from build123d import *

# Parameters (mm, degrees)
SKETCH1_W           = 18
SKETCH1_H           = 6
BOSS_EXTRUDE1_DEPTH = 17.5
SKETCH2_R           = 1.5
CUT_EXTRUDE1_DEPTH  = 20.906029237
FILLET1_R           = 2
BOSS_EXTRUDE2_DEPTH = 3.75
SKETCH4_W           = 4.2
SKETCH4_H           = 4
BOSS_EXTRUDE3_DEPTH = 2.25
SKETCH5_W           = 4.2
SKETCH5_H           = 8.25
CUT_EXTRUDE2_DEPTH  = 1.25
FILLET5_R           = 1
FILLET6_R           = 1.5
FILLET7_R           = 0.75


with BuildPart() as part:
    # Sketch1 → Boss-Extrude1 (new body)
    with BuildSketch(Plane(origin=(0, 0, 0), x_dir=(1, 0, 0), z_dir=(0, 1, 0))):
        Rectangle(SKETCH1_W, SKETCH1_H)
    extrude(amount=BOSS_EXTRUDE1_DEPTH)

    # Sketch2 → Cut-Extrude1 (cut, through all)
    with BuildSketch(Plane(origin=(0, 17.5, 0), x_dir=(1, 0, 0), z_dir=(0, 1, 0))):
        with Locations(Location((-5, 0, 0), (0, 0, 270))):
            Circle(SKETCH2_R)
        with Locations(Location((5, 0, 0), (0, 0, 90))):
            Circle(SKETCH2_R)
    extrude(amount=-CUT_EXTRUDE1_DEPTH, mode=Mode.SUBTRACT)

    # Fillet1
    fillet1_edges = [part.edges().sort_by_distance(p)[0] for p in [
        (9, 8.75, 3),
        (-9, 8.75, 3),
        (-9, 8.75, -3),
        (9, 8.75, -3),
    ]]
    fillet(fillet1_edges, radius=FILLET1_R)

    # Sketch3 → Boss-Extrude2 (add)
    with BuildSketch(Plane(origin=(0, 0, -3), x_dir=(-1, 0, 0), z_dir=(0, 0, -1))):
        Polygon((-3.25, 17.5), (-3.25, 13), (3.25, 13), (3.25, 17.5), (2.1, 17.5), (2.1, 13.5), (-2.1, 13.5), (-2.1, 17.5), align=None)
    extrude(amount=BOSS_EXTRUDE2_DEPTH)

    # Sketch4 → Boss-Extrude3 (add)
    with BuildSketch(Plane(origin=(0, 0, -3), x_dir=(-1, 0, 0), z_dir=(0, 0, -1))):
        with Locations((0, 15.5)):
            Rectangle(SKETCH4_W, SKETCH4_H)
    extrude(amount=BOSS_EXTRUDE3_DEPTH)

    # Sketch5 → Cut-Extrude2 (cut)
    with BuildSketch(Plane(origin=(0, 17.5, 0), x_dir=(1, 0, 0), z_dir=(0, 1, 0))):
        with Locations((0, 1.125)):
            Rectangle(SKETCH5_W, SKETCH5_H)
    extrude(amount=-CUT_EXTRUDE2_DEPTH, mode=Mode.SUBTRACT)

    # Fillet5
    fillet5_edges = [part.edges().sort_by_distance(p)[0] for p in [
        (0, 16.25, 3),
        (0, 16.25, -5.25),
    ]]
    fillet(fillet5_edges, radius=FILLET5_R)

    # Fillet6
    fillet6_edges = [part.edges().sort_by_distance(p)[0] for p in [
        (0, 13, -3),
        (-3.25, 15.25, -3),
        (3.25, 15.25, -3),
    ]]
    fillet(fillet6_edges, radius=FILLET6_R)

    # Fillet7
    # the kernel refuses this fillet: 0.75 mm, written as the material it takes off along each edge
    with BuildSketch(Plane(origin=(5.125, 13, -6.75), x_dir=(0, 1, 0), z_dir=(-1, 0, 0))) as fillet7_piece_1:
        with BuildLine():
            CenterArc((FILLET7_R, -FILLET7_R), FILLET7_R, 90, 90)
            Line((0, -FILLET7_R), (0, 0))
            Line((0, 0), (FILLET7_R, 0))
        make_face()
    extrude(amount=10.25, mode=Mode.SUBTRACT)


solid = part.part
Geometry: final body of the model. Coordinates: model frame, mm. A direction names the side the tool comes from. Round coordinates to 2 decimals unless told otherwise and drop trailing zeros. Loops run counter-clockwise (first coordinate to the right, second up) from the corner with the lowest first, then second, coordinate; pieces in that order, holes last. Notation, with made-up numbers: M -7,56 L 39,56 A28 ccw 39,76 Z; hole C 41.5,79 d5. An arc over 180 degrees is marked long. One line per question, with ' | ' between items.
(1) Pull-direction query (X, two-part tool) for faces 4 (the cylindrical face through (-8.43, 8.87, 2.4)), 5 (the flat face through (0, 13, -5)), 6 (the flat face through (0, 13.5, -6)); classes: +X half, -X half, draft (parallel to the pull), parting line (faces both ways), or undercut.
Check result:
face 4: -X half | face 5: draft | face 6: undercut
(2) Cut plane C-C on z = 0. Return the cut outline in (x, y), plus the area to 3 significant figures.
Check result:
outline: M -9,0 L -6.5,0 L -6.5,17.5 L -9,17.5 Z; M -3.5,0 L 3.5,0 L 3.5,17.5 L 2.1,17.5 L 2.1,16.25 L -2.1,16.25 L -2.1,17.5 L -3.5,17.5 Z; M 6.5,0 L 9,0 L 9,17.5 L 6.5,17.5 Z | area: 205 mm2
(3) Cut plane A-A on x = -5. Return the cut outline in (y, z).
Check result:
outline: M 0,-3 L 17.5,-3 L 17.5,-1.5 L 0,-1.5 Z; M 0,1.5 L 17.5,1.5 L 17.5,3 L 0,3 Z
(4) Material intervals for line 1 along X through (y, z) = (4, 0); line 2 along Z through (x, y) = (5, 5.5); line 3 along X through (y, z) = (15.25, -0.5), sorted ascending. Write a range as from..to.
Check result:
line 1: x = -9..-6.5, -3.5..3.5, 6.5..9 | line 2: z = -3..-1.5, 1.5..3 | line 3: x = -9..-6.41, -3.59..3.59, 6.41..9
(5) Cut plane B-B on y = 14.5. Return the cut outline in (x, z).
Check result:
outline: M -9,-1 A2 ccw -7,-3 L -4.75,-3 A1.5 cw -3.25,-4.5 L -3.25,-6.75 L -2.1,-6.75 L -2.1,-5.25 L 2.1,-5.25 L 2.1,-6.75 L 3.25,-6.75 L 3.25,-4.5 A1.5 cw 4.75,-3 L 7,-3 A2 ccw 9,-1 L 9,1 A2 ccw 7,3 L -7,3 A2 ccw -9,1 Z; hole C -5,0 d3; hole C 5,0 d3
(6) Contact query for flat-ended pins moving along their axis: P1, Ø2.5, axis at y = 15.5, z = -5, coming from the -X side; P2, Ø2.5, axis at x = -5, z = 0, coming from the +Y side; P3, Ø8, axis at x = -1.5, y = 5.5, coming from the -Z side; P4, Ø0.8, axis at x = -0.5, z = -5.5, coming from the -Y side. Output: stop coordinate, or through.
Check result:
P1: stops at x = -3.45 | P2: passes through | P3: stops at z = -3 | P4: stops at y = 13
(7) Cut plane D-D on y = 7. Return the cut outline in (x, z).
Check result:
outline: M -9,-1 A2 ccw -7,-3 L 7,-3 A2 ccw 9,-1 L 9,1 A2 ccw 7,3 L -7,3 A2 ccw -9,1 Z; hole C -5,0 d3; hole C 5,0 d3
(8) Access query for faces 1 (the cylindrical face through (0.029, 15.965, 2.699)), 2 (the flat face through (0, 16.25, -1)), 3 (the cylindrical face through (0.029, 15.965, -4.949)). Directions: +Z, -Z, +X, -X, +Y, -Y. A direction counts if a zero-diameter tool reaches every point of the face in a straight line with its end or side. Return the directions, or none.
Check result:
face 1: +Z, +Y | face 2: +Z, -Z, +Y | face 3: -Z, +Y
